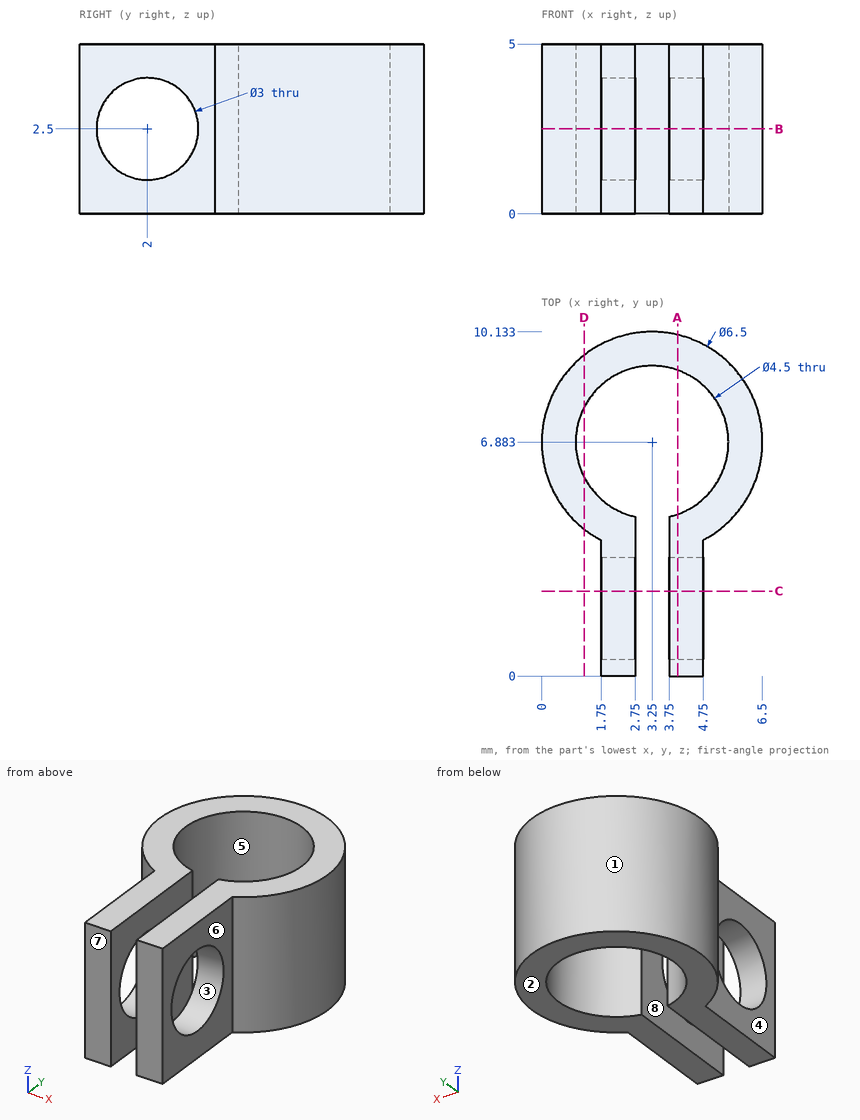
Source: three-view drawing plus pictorial views. Frame: mm from the lowest corner of the part. A direction names the side the tool comes from. Round coordinates to 2 decimals unless told otherwise and drop trailing zeros. Loops run counter-clockwise (first coordinate to the right, second up) from the corner with the lowest first, then second, coordinate; pieces in that order, holes last.
1. Section query A-A on x = 4. Output: boundary loops of the cut face in (y, z).
2. Section query B-B on z = 2.5. Output: boundary loops of the cut face in (x, y).
3. Mould query, pull axis Y, two halves, no side actions, for the marked faces 1, 2 and 3. Classes: released by +Y, released by -Y, zero draft, split by the parting line, or undercut.
4. Ray query, L1, parallel to X at y = 0.5, z = 4.25; L2, parallel to Z at x = 4.45, y = 2; L3, parallel to Y at x = 4, z = 2.55 (1 decimal). Return the intervals inside material, ascending.
5. Section query D-D on x = 1.25. Output: boundary loops of the cut face in (y, z) (1 decimal), and give its area (3 significant figures).
6. Section query C-C on y = 2.5. Output: boundary loops of the cut face in (x, z).
7. Contact query for a flat-ended pin moving along its axis: pin 1 (2.5 mm diameter, centred on y = 1.5, z = 1.5, fed in from -X). Output: stop coordinate, or through.
8. Access query for the marked faces 4, 5, 6, 7 and 8. Directions: +Z, -Z, +X, -X, +Y, -Y. A direction counts if a zero-diameter tool reaches every point of the face in a straight line with its end or side. Return the directions, or none.
Answers below:
1. outline: (0, 0) - (4.76, 0) - (4.76, 5) - (0, 5) - close; (9, 0) - (10.05, 0) - (10.05, 5) - (9, 5) - close; hole circle Ø3 at (2, 2.5)
2. outline: (1.75, 0) - (2.75, 0) - (2.75, 0.5) - (1.75, 0.5) - close; (1.75, 3.5) - (2.75, 3.5) - (2.75, 4.69) arc R2.25 cw (long way) to (3.75, 4.69) - (3.75, 3.5) - (4.75, 3.5) - (4.75, 4) arc R3.25 ccw (long way) to (1.75, 4) - close; (3.75, 0) - (4.75, 0) - (4.75, 0.5) - (3.75, 0.5) - close
3. face 1: split by the parting line
3. face 2: zero draft
3. face 3: undercut
4. L1: x = 1.75 to 2.75, 3.75 to 4.75
4. L2: z = 0 to 1, 4 to 5
4. L3: y = 0 to 0.5, 3.5 to 4.8, 9 to 10
5. outline: (4.3, 0) - (5.9, 0) - (5.9, 5) - (4.3, 5) - close; (7.9, 0) - (9.4, 0) - (9.4, 5) - (7.9, 5) - close
5. area: 15.3 mm2
6. outline: (1.75, 0) - (2.75, 0) - (2.75, 1.09) - (1.75, 1.09) - close; (1.75, 3.91) - (2.75, 3.91) - (2.75, 5) - (1.75, 5) - close; (3.75, 0) - (4.75, 0) - (4.75, 1.09) - (3.75, 1.09) - close; (3.75, 3.91) - (4.75, 3.91) - (4.75, 5) - (3.75, 5) - close
7. pin 1: stops at x = 1.75
8. face 4: +Z, -Z, -X, -Y
8. face 5: +Z, -Z
8. face 6: +Z, -Z, +X, -Y
8. face 7: +Z, -Z, +X, -X, -Y
8. face 8: +Z, -Z, -Y
